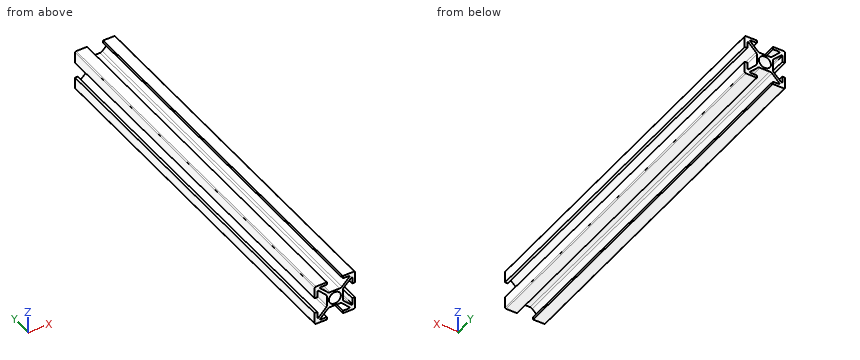
from build123d import *

# Parameters (mm, degrees)
ESBO_O1_R                = 3
RESSALTO_EXTRUS_O1_DEPTH = 188


with BuildPart() as part:
    # Esboço1 → Ressalto-extrusão1 (new body)
    with BuildSketch(Plane(origin=(0, 0, 0), x_dir=(1, 0, 0), z_dir=(0, 1, 0))):
        with BuildLine():
            Line((-7.056497116, 8.7), (-4, 8.7))
            Line((-4, 8.7), (-4, 10))
            Line((-4, 10), (-9.5, 10))
            ThreePointArc((-9.5, 10), (-9.853553391, 9.853553391), (-10, 9.5))
            Line((-10, 9.5), (-10, 4))
            Line((-10, 4), (-8.7, 4))
            Line((-8.7, 4), (-8.7, 7.056497116))
            ThreePointArc((-8.7, 7.056497116), (-8.51480503, 7.333660975), (-8.187867966, 7.26862915))
            Line((-8.187867966, 7.26862915), (-4.439339828, 3.520101013))
            ThreePointArc((-4.439339828, 3.520101013), (-4.114180701, 3.033465989), (-4, 2.459440841))
            Line((-4, 2.459440841), (-4, -2.459440841))
            ThreePointArc((-4, -2.459440841), (-4.114180701, -3.033465989), (-4.439339828, -3.520101013))
            Line((-4.439339828, -3.520101013), (-8.187867966, -7.26862915))
            ThreePointArc((-8.187867966, -7.26862915), (-8.51480503, -7.333660975), (-8.7, -7.056497116))
            Line((-8.7, -7.056497116), (-8.7, -4))
            Line((-8.7, -4), (-10, -4))
            Line((-10, -4), (-10, -9.5))
            ThreePointArc((-10, -9.5), (-9.853553391, -9.853553391), (-9.5, -10))
            Line((-9.5, -10), (-4, -10))
            Line((-4, -10), (-4, -8.7))
            Line((-4, -8.7), (-7.056497116, -8.7))
            ThreePointArc((-7.056497116, -8.7), (-7.333660975, -8.51480503), (-7.26862915, -8.187867966))
            Line((-7.26862915, -8.187867966), (-3.520101013, -4.439339828))
            ThreePointArc((-3.520101013, -4.439339828), (-3.033465989, -4.114180701), (-2.459440841, -4))
            Line((-2.459440841, -4), (2.459440841, -4))
            ThreePointArc((2.459440841, -4), (3.033465989, -4.114180701), (3.520101013, -4.439339828))
            Line((3.520101013, -4.439339828), (7.26862915, -8.187867966))
            ThreePointArc((7.26862915, -8.187867966), (7.333660975, -8.51480503), (7.056497116, -8.7))
            Line((7.056497116, -8.7), (4, -8.7))
            Line((4, -8.7), (4, -10))
            Line((4, -10), (9.5, -10))
            ThreePointArc((9.5, -10), (9.853553391, -9.853553391), (10, -9.5))
            Line((10, -9.5), (10, -4))
            Line((10, -4), (8.7, -4))
            Line((8.7, -4), (8.7, -7.056497116))
            ThreePointArc((8.7, -7.056497116), (8.51480503, -7.333660975), (8.187867966, -7.26862915))
            Line((8.187867966, -7.26862915), (4.439339828, -3.520101013))
            ThreePointArc((4.439339828, -3.520101013), (4.114180701, -3.033465989), (4, -2.459440841))
            Line((4, -2.459440841), (4, 2.459440841))
            ThreePointArc((4, 2.459440841), (4.114180701, 3.033465989), (4.439339828, 3.520101013))
            Line((4.439339828, 3.520101013), (8.187867966, 7.26862915))
            ThreePointArc((8.187867966, 7.26862915), (8.51480503, 7.333660975), (8.7, 7.056497116))
            Line((8.7, 7.056497116), (8.7, 4))
            Line((8.7, 4), (10, 4))
            Line((10, 4), (10, 9.5))
            ThreePointArc((10, 9.5), (9.853553391, 9.853553391), (9.5, 10))
            Line((9.5, 10), (4, 10))
            Line((4, 10), (4, 8.7))
            Line((4, 8.7), (7.056497116, 8.7))
            ThreePointArc((7.056497116, 8.7), (7.333660975, 8.51480503), (7.26862915, 8.187867966))
            Line((7.26862915, 8.187867966), (3.520101013, 4.439339828))
            ThreePointArc((3.520101013, 4.439339828), (3.033465989, 4.114180701), (2.459440841, 4))
            Line((2.459440841, 4), (-2.459440841, 4))
            ThreePointArc((-2.459440841, 4), (-3.033465989, 4.114180701), (-3.520101013, 4.439339828))
            Line((-3.520101013, 4.439339828), (-7.26862915, 8.187867966))
            ThreePointArc((-7.26862915, 8.187867966), (-7.333660975, 8.51480503), (-7.056497116, 8.7))
        make_face()
        Circle(ESBO_O1_R, mode=Mode.SUBTRACT)
    extrude(amount=RESSALTO_EXTRUS_O1_DEPTH)


solid = part.part
Read the model definition and answer for the solid it produces. Units are mm, in the model's axes. Coordinates: 2 decimals unless noted, no trailing zeros. Loops run counter-clockwise (first coordinate to the right, second up) from the corner with the lowest first, then second, coordinate; pieces in that order, holes last. Notation, with made-up numbers: (-29, -30.5) -> (5, -30.5) arc R23 cw to (5, -0.5) -> close; hole circle Ø3 at (70.25, 67.25). An arc over 180 degrees is marked (long way). Answer in a Markdown table with one row per item.
Item 1: A cutting plane is placed at B-B on z = 0. Determine the outline of the cut face in (x, y), plus the area to 3 significant figures.
Returned:
| item | result |
|---|---|
| outline | (-4, 0) -> (-3, 0) -> (-3, 188) -> (-4, 188) -> close; (3, 0) -> (4, 0) -> (4, 188) -> (3, 188) -> close |
| area | 376 mm^2 |
Item 2: Straight lines are drawn through the part: line 1 along Z through (x, y) = (8.5, 80); line 2 along X through (y, z) = (147, 0). For each, find the intervals that lie inside material, in ascending order. Write a range as [from, to].
Returned:
| item | result |
|---|---|
| line 1 | z = [-10, -7.34], [7.34, 10] |
| line 2 | x = [-4, -3], [3, 4] |
Item 3: A cutting plane is placed at A-A on x = 0. Determine the outline of the cut face in (y, z), plus the area to 3 significant figures.
Returned:
| item | result |
|---|---|
| outline | (0, -4) -> (188, -4) -> (188, -3) -> (0, -3) -> close; (0, 3) -> (188, 3) -> (188, 4) -> (0, 4) -> close |
| area | 376 mm^2 |
Item 4: Each of these flat-tipped pins is pushed along its axis until it touches: P1, Ø4, axis at x = -0.5, y = 137.5, coming from the -Z side; P2, Ø2.5, axis at y = 85.5, z = -1, coming from the +X side; P3, Ø4, axis at x = -1.5, y = 29, coming from the +Z side; P4, Ø3, axis at x = 1, z = 6, coming from the -Y side. Where does it stop, or does it pass through?
Returned:
| item | result |
|---|---|
| P1 | stops at z = -4 |
| P2 | stops at x = 4 |
| P3 | stops at z = 4.42 |
| P4 | passes through |
